Part print with two shaded views. Sizes in mm from the minimum x, y, z corner. Round coordinates to 2 decimals unless told otherwise and drop trailing zeros. Order: outer loops, then holes, each group sorted by start corner. A loop starts at its lowest first (then second) coordinate and runs counter-clockwise, first axis right, second up. Notation, with made-up numbers: M 5.5,-32.75 L 49.5,-32.75 A15 cw 49.5,-27.75 Z; hole C 50,6.25 d2. An arc over 180 degrees is marked long. Put each result on its own line as item: value.
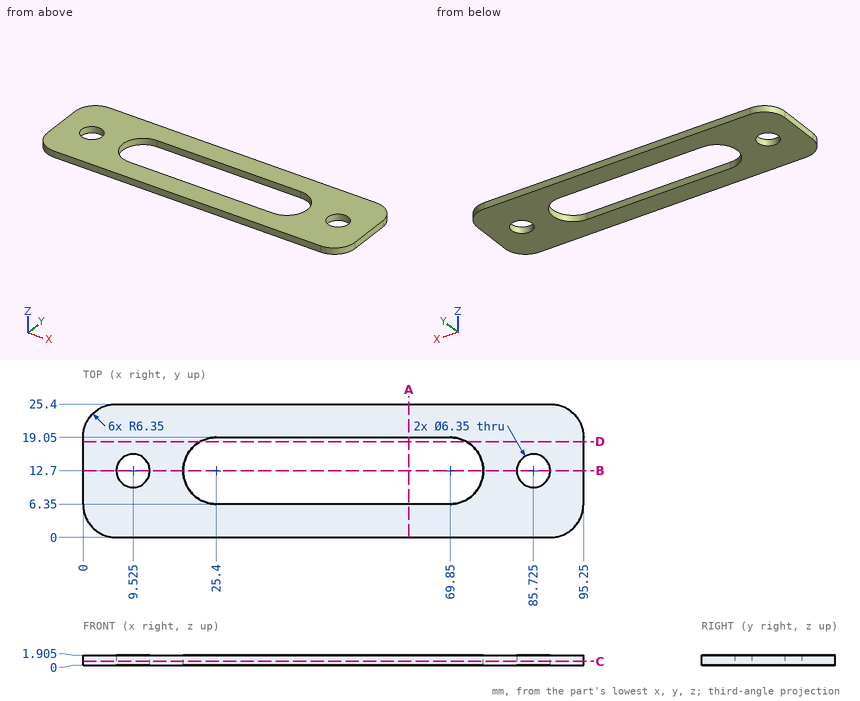
Item 1: Band-saw the part on B-B on y = 12.7. Give the cut face in (x, z) (3 decimals).
Answers below:
outline: M 0,0 L 6.35,0 L 6.35,1.905 L 0,1.905 Z; M 12.7,0 L 19.05,0 L 19.05,1.905 L 12.7,1.905 Z; M 76.2,0 L 82.55,0 L 82.55,1.905 L 76.2,1.905 Z; M 88.9,0 L 95.25,0 L 95.25,1.905 L 88.9,1.905 Z
Item 2: Pin check, flat tip, straight feed: P1, Ø7.5, axis at x = 85.725, y = 12.7, coming from the +Z side (3 decimals). Stop position of the tip, or through.
Answers below:
P1: z = 1.905
Item 3: Band-saw the part on D-D on y = 18.25. Give the cut face in (x, z) (3 decimals).
Answers below:
outline: M 0,0 L 22.315,0 L 22.315,1.905 L 0,1.905 Z; M 72.935,0 L 95.25,0 L 95.25,1.905 L 72.935,1.905 Z
Item 4: Band-saw the part on C-C on z = 0.8. Give the cut face in (x, y) (3 decimals).
Answers below:
outline: M 0,6.35 A6.35 ccw 6.35,0 L 88.9,0 A6.35 ccw 95.25,6.35 L 95.25,19.05 A6.35 ccw 88.9,25.4 L 6.35,25.4 A6.35 ccw 0,19.05 Z; hole C 9.525,12.7 d6.35; hole M 25.4,6.35 L 69.85,6.35 A6.35 ccw 69.85,19.05 L 25.4,19.05 A6.35 ccw Z; hole C 85.725,12.7 d6.35
Item 5: Probe line 1 along Y through (x, z) = (40.5, 1.25); line 2 along X through (y, z) = (13.75, 1.7); line 3 along X through (y, z) = (10.5, 0.5). List the from-to ranges inside material, lowest first. Write a range as [from, to].
Answers below:
line 1: [0, 6.35], [19.05, 25.4]
line 2: [0, 6.53], [12.52, 19.14], [76.11, 82.73], [88.72, 95.25]
line 3: [0, 7.24], [11.81, 19.44], [75.81, 83.44], [88.01, 95.25]
Item 6: Band-saw the part on A-A on x = 62. Give the cut face in (y, z) (3 decimals), and give its area (3 significant figures).
Answers below:
outline: M 0,0 L 6.35,0 L 6.35,1.905 L 0,1.905 Z; M 19.05,0 L 25.4,0 L 25.4,1.905 L 19.05,1.905 Z
area: 24.2 mm²
